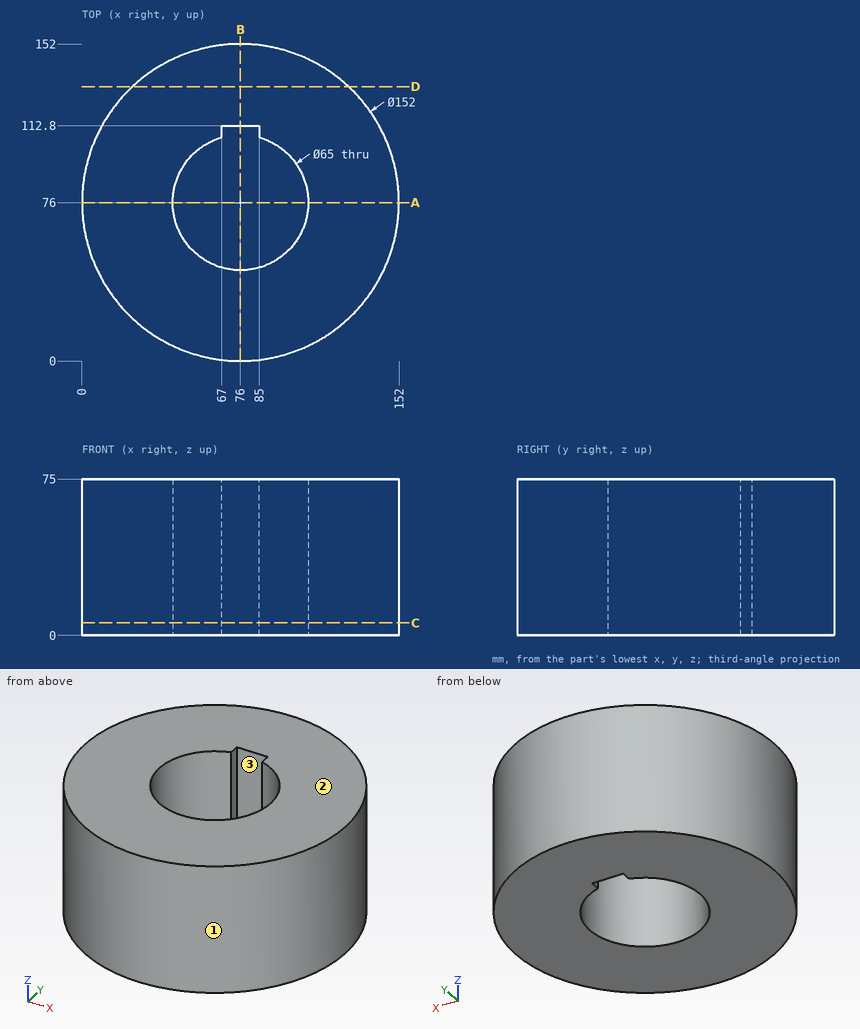
Design review of the part shown in the three views and the two pictorial views. Dimensions are in mm from the part's minimum x, y and z. Coordinates: 2 decimals unless noted, no trailing zeros. Write each loop counter-clockwise with the first axis right and the second up, starting at its lowest first coordinate (ties: lowest second). Pieces come first, ordered by that corner, then holes.
(1) Wall thickness on probe 1 along Y at (x, z) = (76, 18); probe 2 along Y at (x, z) = (92, 57.5); probe 3 along X at (y, z) = (82.5, 8): over which ranges is each line inside the solid? List them lowest first.
(2) For pin 1 Ø2 at (y, z) = (79.5, 15.5) entering from +X; pin 2 Ø12 at (y, z) = (127, 39) entering from +X; pin 3 Ø3 at (y, z) = (45.5, 52) entering from -X; pin 4 Ø8 at (x, y) = (74, 49.5) entering from +Z (3 decimals), all flat-tipped, find the tip position at first contact; note any pin that passes through.
(3) Add section D-D on y = 131.5. Give the boundary of the cut face in (x, z).
(4) Add section C-C on z = 6. Give the boundary of the cut face in (x, y), then the cut area to 3 significant figures.
(5) Add section B-B on x = 76. Give the boundary of the cut face in (y, z), then the cut area to 3 significant figures.
(6) Add section A-A on y = 76. Give the boundary of the cut face in (x, z), then the cut area to 4 significant figures.
(7) The part is to be moulded in two halves that separate along Y. For the marked faces 1, 2 and 3, say which applies: +Y half, -Y half, draft (parallel to the pull), parting line (faces both ways), or undercut.
Answer sheet:
1. probe 1: y = 0 to 43.5, 112.8 to 152
1. probe 2: y = 1.7 to 47.71, 104.29 to 150.3
1. probe 3: x = 0.28 to 44.16, 107.84 to 151.72
2. pin 1: stops at x = 151.96
2. pin 2: stops at x = 137.25
2. pin 3: stops at x = 5.75
2. pin 4: passes through
3. outline: (24.08, 0) - (127.92, 0) - (127.92, 75) - (24.08, 75) - close
4. outline: circle Ø152 at (76, 76); hole (67, 107.23) arc R32.5 ccw (long way) to (85, 107.23) - (85, 112.8) - (67, 112.8) - close
4. area: 14,700 mm2
5. outline: (0, 0) - (43.5, 0) - (43.5, 75) - (0, 75) - close; (112.8, 0) - (152, 0) - (152, 75) - (112.8, 75) - close
5. area: 6,200 mm2
6. outline: (0, 0) - (43.5, 0) - (43.5, 75) - (0, 75) - close; (108.5, 0) - (152, 0) - (152, 75) - (108.5, 75) - close
6. area: 6,525 mm2
7. face 1: parting line
7. face 2: draft
7. face 3: undercut
